Source: CAD feature listing. Evaluate the final solid. Frame: model axes, mm. Coordinates: 2 decimals unless noted, no trailing zeros. Order: outer loops, then holes, each group sorted by start corner. A loop starts at its lowest first (then second) coordinate and runs counter-clockwise, first axis right, second up.
```python
from build123d import *

# Parameters (mm, degrees)
BOSS_EXTRUDE1_DEPTH = 1.5875
SKETCH2_W           = 31.75
SKETCH2_H           = 3.175
SKETCH2_W_2         = 12.7
CUT_EXTRUDE1_DEPTH  = 3.175


with BuildPart() as part:
    # Sketch1 → Boss-Extrude1 (new, symmetric)
    with BuildSketch(Plane.XY):
        Polygon((-76.2, 82.55), (-76.2, 69.85), (-79.375, 69.85), (-79.375, 57.15), (-76.2, 57.15), (-76.2, 44.45), (-79.375, 44.45), (-79.375, 31.75), (-76.2, 31.75), (-76.2, 19.05), (-79.375, 19.05), (-79.375, 6.35), (-76.2, 6.35), (-76.2, -6.35), (-79.375, -6.35), (-79.375, -19.05), (-76.2, -19.05), (-76.2, -31.75), (-79.375, -31.75), (-79.375, -44.45), (-76.2, -44.45), (-76.2, -57.15), (-79.375, -57.15), (-79.375, -69.85), (-76.2, -69.85), (-76.2, -82.55), (76.2, -82.55), (76.2, -69.85), (79.375, -69.85), (79.375, -57.15), (76.2, -57.15), (76.2, -44.45), (79.375, -44.45), (79.375, -31.75), (76.2, -31.75), (76.2, -19.05), (79.375, -19.05), (79.375, -6.35), (76.2, -6.35), (76.2, 6.35), (79.375, 6.35), (79.375, 19.05), (76.2, 19.05), (76.2, 31.75), (79.375, 31.75), (79.375, 44.45), (76.2, 44.45), (76.2, 57.15), (79.375, 57.15), (79.375, 69.85), (76.2, 69.85), (76.2, 82.55), align=None)
    extrude(amount=BOSS_EXTRUDE1_DEPTH, both=True)

    # Sketch2 → Cut-Extrude1 (cut)
    with BuildSketch(Plane(origin=(0, 82.55, 0), x_dir=(1, 0, 0), z_dir=(0, 1, 0))):
        with Locations((60.325, 0)):
            Rectangle(SKETCH2_W, SKETCH2_H)
        with Locations((-60.325, 0)):
            Rectangle(SKETCH2_W, SKETCH2_H)
        with Locations((25.4, 0)):
            Rectangle(SKETCH2_W_2, SKETCH2_H)
        Rectangle(SKETCH2_W_2, SKETCH2_H)
        with Locations((-25.4, 0)):
            Rectangle(SKETCH2_W_2, SKETCH2_H)
    extrude(amount=-CUT_EXTRUDE1_DEPTH, mode=Mode.SUBTRACT)


solid = part.part
```
Q1. Material intervals for line 1 along Y through (x, z) = (58, -0.4) (3 decimals); line 2 along X through (y, z) = (-1, 0.15), sorted ascending.
Solutions:
line 1: y = -82.55 to 79.375
line 2: x = -76.2 to 76.2
Q2. Pin query (flat end, axial travel): P1, Ø1.6, axis at y = 0, z = -0.5, coming from the -X side; P2, Ø1.6, axis at y = -50, z = 0, coming from the +X side; P3, Ø1, axis at x = 78.5, z = 0, coming from the +Y side. Return the tip coordinate at first contact, or that it passes through.
Solutions:
P1: stops at x = -76.2
P2: stops at x = 76.2
P3: stops at y = 69.85
Q3. Section query A-A on y = 51. Output: boundary loops of the cut face in (x, z).
Solutions:
outline: (-76.2, -1.59) - (76.2, -1.59) - (76.2, 1.59) - (-76.2, 1.59) - close
